Geometry check sheet. Reference: the model listing, model coordinates, mm. Face numbers are marked on the shaded views. Give positions to 0.01 mm unless a question says otherwise; leave off trailing zeros. Loops run counter-clockwise (first coordinate to the right, second up) from the corner with the lowest first, then second, coordinate; pieces in that order, holes last. Notation, with made-up numbers: (9.5, 73) -> (37.5, 73) arc R14 ccw to (37.5, 82) -> close; hole circle Ø2 at (25.25, 25). An arc over 180 degrees is marked (long way). Answer in a Markdown table with one row per item. Add a question column.
```python
from build123d import *

# Parameters (mm, degrees)
SKETCH1_R           = 25
BOSS_EXTRUDE1_DEPTH = 5
SKETCH2_R           = 5
CUT_EXTRUDE1_DEPTH  = 6
CIRPATTERN1_COUNT   = 12
SKETCH3_R           = 4
CUT_EXTRUDE2_DEPTH  = 6
SKETCH4_R           = 1.5
CUT_EXTRUDE3_DEPTH  = 6


with BuildPart() as part:
    # Sketch1 → Boss-Extrude1 (new body)
    with BuildSketch(Plane(origin=(0, 0, 0), x_dir=(1, 0, 0), z_dir=(0, 1, 0))):
        Circle(SKETCH1_R)
    extrude(amount=BOSS_EXTRUDE1_DEPTH)

    # Sketch2 → Cut-Extrude1 (cut, through all)
    with BuildSketch(Plane(origin=(0, 0, 0), x_dir=(1, 0, 0), z_dir=(0, 1, 0))):
        with Locations((0, 28.5)):
            Circle(SKETCH2_R)
    cut_extrude1 = extrude(amount=CUT_EXTRUDE1_DEPTH, mode=Mode.SUBTRACT)

    # CirPattern1: Cut-Extrude1 ×12 about axis
    cirpattern1_axis = Axis((0, 0, 0), (0, 1, 0))
    for i in range(1, CIRPATTERN1_COUNT):
        add(cut_extrude1.rotate(cirpattern1_axis, i * 360 / CIRPATTERN1_COUNT), mode=Mode.SUBTRACT)

    # Sketch3 → Cut-Extrude2 (cut, through all)
    with BuildSketch(Plane(origin=(0, 0, 0), x_dir=(1, 0, 0), z_dir=(0, 1, 0))):
        Circle(SKETCH3_R)
    extrude(amount=CUT_EXTRUDE2_DEPTH, mode=Mode.SUBTRACT)

    # Sketch4 → Cut-Extrude3 (cut, through all)
    with BuildSketch(Plane(origin=(0, 5, 0), x_dir=(1, 0, 0), z_dir=(0, 1, 0))):
        with Locations((-12, 0)):
            Circle(SKETCH4_R)
        with Locations((12, 0)):
            Circle(SKETCH4_R)
    extrude(amount=-CUT_EXTRUDE3_DEPTH, mode=Mode.SUBTRACT)


solid = part.part
```
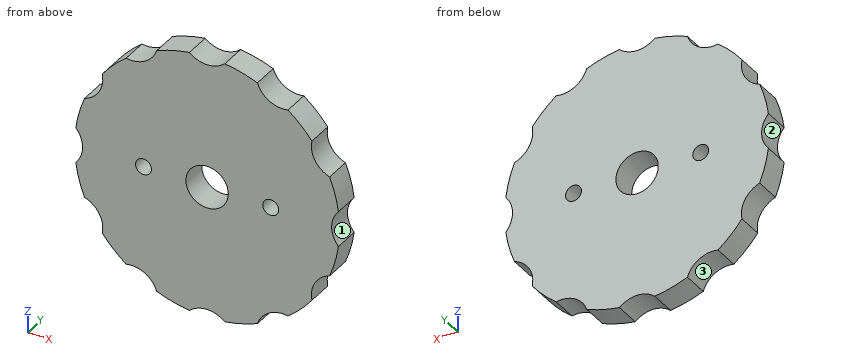
1. Material ranges on L1, parallel to X at y = 2.35, z = 0; L2, parallel to Z at x = 14, y = 4.45; L3, parallel to Z at x = 0, y = 3.95, recorded low to high. Write a range as from..to.
2. Sectioned sample at D-D (x = -12). Enter the section's corners in (y, z), plus the area to 3 significant figures.
3. Release check for a two-part mould opening along X. For the marked faces 1, 2 and 3 record: released by +X, released by -X, zero draft, split by the parting line, or undercut.
4. Sectioned sample at A-A (z = 0). Enter the section's corners in (x, y).
5. Sectioned sample at B-B (x = 0). Enter the section's corners in (y, z), plus the area to 3 significant figures.
6. Sectioned sample at C-C (y = 1.8). Enter the section's corners in (x, z).
7. Gauge pin test, flat ends, axial feed: pin 1 Ø3 at (x, y) = (-5.5, 3.5) entering from -Z; pin 2 Ø2 at (x, y) = (-14.5, 1.5) entering from +Z. Record the tip position at first contact, or that the pin passes through.
Response:
| question | item | result |
|---|---|---|
| 1 | L1 | x = -23.5..-13.5, -10.5..-4, 4..10.5, 13.5..23.5 |
| 1 | L2 | z = -19.69..19.69 |
| 1 | L3 | z = -23.5..-4, 4..23.5 |
| 2 | outline | (0, -20.22) -> (5, -20.22) -> (5, -1.5) -> (0, -1.5) -> close; (0, 1.5) -> (5, 1.5) -> (5, 20.22) -> (0, 20.22) -> close |
| 2 | area | 187 mm2 |
| 3 | face 1 | released by +X |
| 3 | face 2 | released by -X |
| 3 | face 3 | undercut |
| 4 | outline | (-23.5, 0) -> (-13.5, 0) -> (-13.5, 5) -> (-23.5, 5) -> close; (-10.5, 0) -> (-4, 0) -> (-4, 5) -> (-10.5, 5) -> close; (4, 0) -> (10.5, 0) -> (10.5, 5) -> (4, 5) -> close; (13.5, 0) -> (23.5, 0) -> (23.5, 5) -> (13.5, 5) -> close |
| 5 | outline | (0, -23.5) -> (5, -23.5) -> (5, -4) -> (0, -4) -> close; (0, 4) -> (5, 4) -> (5, 23.5) -> (0, 23.5) -> close |
| 5 | area | 195 mm2 |
| 6 | outline | (-24.78, -3.34) arc R25 ccw to (-23.13, -9.5) arc R5 cw to (-19.79, -15.28) arc R25 ccw to (-15.28, -19.79) arc R5 cw to (-9.5, -23.13) arc R25 ccw to (-3.34, -24.78) arc R5 cw to (3.34, -24.78) arc R25 ccw to (9.5, -23.13) arc R5 cw to (15.28, -19.79) arc R25 ccw to (19.79, -15.28) arc R5 cw to (23.13, -9.5) arc R25 ccw to (24.78, -3.34) arc R5 cw to (24.78, 3.34) arc R25 ccw to (23.13, 9.5) arc R5 cw to (19.79, 15.28) arc R25 ccw to (15.28, 19.79) arc R5 cw to (9.5, 23.13) arc R25 ccw to (3.34, 24.78) arc R5 cw to (-3.34, 24.78) arc R25 ccw to (-9.5, 23.13) arc R5 cw to (-15.28, 19.79) arc R25 ccw to (-19.79, 15.28) arc R5 cw to (-23.13, 9.5) arc R25 ccw to (-24.78, 3.34) arc R5 cw to start; hole circle Ø3 at (-12, 0); hole circle Ø8 at (0, 0); hole circle Ø3 at (12, 0) |
| 7 | pin 1 | stops at z = -24.68 |
| 7 | pin 2 | stops at z = 19.79 |
